```python
from build123d import *

# Parameters (mm, degrees)
SKETCH1_R           = 4
BOSS_EXTRUDE1_DEPTH = 10
SCALE1_SCALE        = 0.5


with BuildPart() as part:
    # Sketch1 → Boss-Extrude1 (new body)
    with BuildSketch(Plane(origin=(0, 0, 0), x_dir=(1, 0, 0), z_dir=(0, 1, 0))):
        with BuildLine():
            Line((-28.284271247, 28.284271247), (-28.284271247, -48.415659381))
            Line((-28.284271247, -48.415659381), (63.338627893, -48.415659381))
            Line((63.338627893, -48.415659381), (68.284271247, -48.415659381))
            Line((68.284271247, -48.415659381), (68.284271247, 28.284271247))
            Line((68.284271247, 28.284271247), (108.284271247, 28.284271247))
            ThreePointArc((108.284271247, 28.284271247), (133.284271247, 53.284271247), (108.284271247, 78.284271247))
            Line((108.284271247, 78.284271247), (68.284271247, 78.284271247))
            Line((68.284271247, 78.284271247), (35, 115.595895274))
            Line((35, 115.595895274), (5, 115.595895274))
            Line((5, 115.595895274), (-28.284271247, 78.284271247))
            Line((-28.284271247, 78.284271247), (-73.439346791, 78.284271247))
            Line((-73.439346791, 78.284271247), (-73.439346791, 28.284271247))
            Line((-73.439346791, 28.284271247), (-28.284271247, 28.284271247))
        make_face()
        with Locations((5, 100)):
            Circle(SKETCH1_R, mode=Mode.SUBTRACT)
        with Locations((35, 100)):
            Circle(SKETCH1_R, mode=Mode.SUBTRACT)
        with Locations((-13.284271247, 53.284271247)):
            Circle(SKETCH1_R, mode=Mode.SUBTRACT)
        with BuildLine():
            Line((53.284271247, 68.284271247), (83.284271247, 68.284271247))
            ThreePointArc((83.284271247, 68.284271247), (98.284271247, 53.284271247), (83.284271247, 38.284271247))
            Line((83.284271247, 38.284271247), (53.284271247, 38.284271247))
            ThreePointArc((53.284271247, 38.284271247), (38.284271247, 53.284271247), (53.284271247, 68.284271247))
        make_face(mode=Mode.SUBTRACT)
    extrude(amount=BOSS_EXTRUDE1_DEPTH)


with BuildPart() as part_1:
    # Scale1: scaled about (19.875908693, 5, -32.344377814)
    add(part.part.scale(SCALE1_SCALE).moved(Location((9.937954346, 2.5, -16.172188907))))


solid = part_1.part
```
Geometry: final body of the model. Coordinates: model frame, mm. A direction names the side the tool comes from. Round coordinates to 2 decimals unless told otherwise and drop trailing zeros. Order: outer loops, then holes, each group sorted by start corner. A loop starts at its lowest first (then second) coordinate and runs counter-clockwise, first axis right, second up. Notation, with made-up numbers: (-27.5, 89.5) - (28.5, 89.5) arc R20 ccw to (28.5, 115.5) - close; hole circle Ø5 at (20, -33). An arc over 180 degrees is marked (long way). Write item = value, one per line. Start each with the question number.
Q1. Cut plane D-D on x = 68. Return the cut outline in (y, z), and give its area (3 significant figures).
Q2. Cut plane A-A on x = 41. Return the cut outline in (y, z).
Q3. Cut plane B-B on y = 5.45. Return the cut outline in (x, z), and give its area (3 significant figures).
Q4. Access query for faces 4 (the flat face through (-15, 5, -55.314)), 5 (the flat face through (-4.204, 5, -11)), 6 (the flat face through (54, 5, -30.314)). Directions: +Z, -Z, +X, -X, +Y, -Y. A direction counts if a zero-diameter tool reaches every point of the face in a straight line with its end or side. Return the directions, or none.
Q5. Pull-direction query (Z, two-part tool) for faces 1 (the flat face through (44, 5, -50.314)), 2 (the flat face through (20, 5, -73.97)), 3 (the flat face through (24, 2.5, -34)); classes: +Z half, -Z half, draft (parallel to the pull), parting line (faces both ways), or undercut.
Q6. Ray query, line 1 (Z direction, x = 46.5, y = 2.8); line 2 (X direction, y = 5, z = -43.5); line 3 (X direction, y = 4.95, z = -8). Return the intervals inside material, ascending. Write a range as from..to.
Q7. Cut plane C-C on z = -14. Return the cut outline in (x, y), and give its area (3 significant figures).
Q8. Pin query (flat end, axial travel): pin 1 (2 mm diameter, centred on x = 43, y = 3, fed in from -Z); pin 2 (1.5 mm diameter, centred on x = 49.5, y = 6, fed in from +Z); pin 3 (3.5 mm diameter, centred on x = 3.3, z = -42.81, fed in from -Y); pin 4 (1.5 mm diameter, centred on x = 43, y = 4.5, fed in from -Z). Return the tip coordinate at first contact, or that it passes through.
Outcome:
q1.outline = (2.5, -54.68) - (7.5, -54.68) - (7.5, -30.94) - (2.5, -30.94) - close
q1.area = 119 mm^2
q2.outline = (2.5, -58.77) - (7.5, -58.77) - (7.5, -50.31) - (2.5, -50.31) - close; (2.5, -35.31) - (7.5, -35.31) - (7.5, 8.04) - (2.5, 8.04) - close
q3.outline = (-26.78, -55.31) - (-4.2, -55.31) - (12.44, -73.97) - (27.44, -73.97) - (44.08, -55.31) - (64.08, -55.31) arc R12.5 ccw to (64.08, -30.31) - (44.08, -30.31) - (44.08, 8.04) - (-4.2, 8.04) - (-4.2, -30.31) - (-26.78, -30.31) - close; hole circle Ø4 at (3.3, -42.81); hole circle Ø4 at (12.44, -66.17); hole circle Ø4 at (27.44, -66.17); hole (36.58, -50.31) - (51.58, -50.31) arc R7.5 ccw to (51.58, -35.31) - (36.58, -35.31) arc R7.5 ccw to start
q3.area = 4,520 mm^2
q4.face_4 = -Z, -X, +Y, -Y
q4.face_5 = +Z, -X, +Y, -Y
q4.face_6 = +Z, +X, +Y, -Y
q5.face_1 = undercut
q5.face_2 = -Z half
q5.face_3 = draft
q6.line_1 = -55.31..-50.31, -35.31..-30.31
q6.line_2 = -26.78..1.42, 5.17..29.11, 59.05..76.56
q6.line_3 = -4.2..44.08
q7.outline = (-4.2, 2.5) - (44.08, 2.5) - (44.08, 7.5) - (-4.2, 7.5) - close
q7.area = 241 mm^2
q8.pin_1 = -57.65
q8.pin_2 = -30.31
q8.pin_3 = through
q8.pin_4 = -57.37
